Model file for the job. Use its own axes, mm. Face numbers are marked on the shaded views. A direction names the side the tool comes from. Round coordinates to 2 decimals unless told otherwise and drop trailing zeros. Loops run counter-clockwise (first coordinate to the right, second up) from the corner with the lowest first, then second, coordinate; pieces in that order, holes last. Notation, with made-up numbers: (66, -22) -> (118, -22) arc R22 cw to (118, 9) -> close; hole circle Ø5 at (20.5, 75.25). An arc over 180 degrees is marked (long way). Use a Markdown table: item, result.
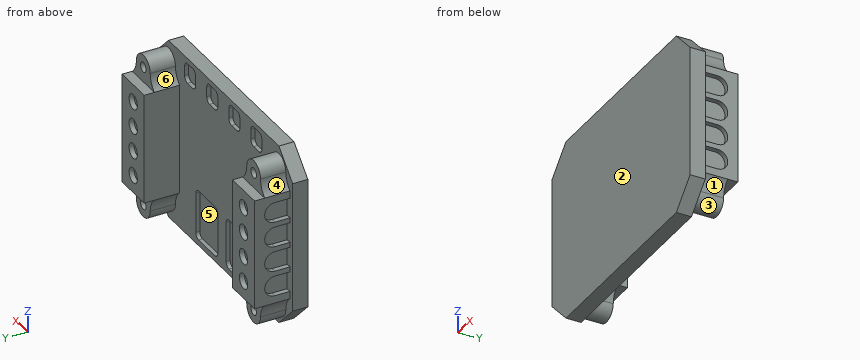
from build123d import *

# Parameters (mm, degrees)
SALIENTE_EXTRUIR1_DEPTH = 3
CROQUIS2_R              = 1
SALIENTE_EXTRUIR2_DEPTH = 7
CROQUIS3_W              = 8.584431172
CROQUIS3_H              = 6.245278734
CROQUIS3_W_2            = 9.103782271
CROQUIS3_H_2            = 6.523642819
CORTAR_EXTRUIR1_DEPTH   = 2
CROQUIS4_R              = 1.5
CORTAR_EXTRUIR2_DEPTH   = 1
CORTAR_EXTRUIR3_DEPTH   = 1
CORTAR_EXTRUIR4_DEPTH   = 0.8


with BuildPart() as part:
    # Croquis1 → Saliente-Extruir1 (new body)
    with BuildSketch(Plane(origin=(0, 0, 0), x_dir=(1, 0, 0), z_dir=(0, 1, 0))):
        Polygon((-25, -13), (-20, -18), (20, -18), (25, -13), (25, 13), (20, 18), (-20, 18), (-25, 13), align=None)
    extrude(amount=SALIENTE_EXTRUIR1_DEPTH)

    # Croquis2 → Saliente-Extruir2 (add)
    with BuildSketch(Plane(origin=(0, 3, 0), x_dir=(1, 0, 0), z_dir=(0, 1, 0))):
        with BuildLine():
            Line((-24, 11), (-24, -11))
            ThreePointArc((-24, -11), (-22.910217487, -12.356554061), (-22.499549169, -14.047475815))
            ThreePointArc((-22.499549169, -14.047475815), (-20, -16.5), (-17.500450831, -14.047475815))
            ThreePointArc((-17.500450831, -14.047475815), (-17.089782513, -12.356554061), (-16, -11))
            Line((-16, -11), (-16, 11))
            ThreePointArc((-16, 11), (-17.089782513, 12.356554061), (-17.500450831, 14.047475815))
            ThreePointArc((-17.500450831, 14.047475815), (-20, 16.5), (-22.499549169, 14.047475815))
            ThreePointArc((-22.499549169, 14.047475815), (-22.910217487, 12.356554061), (-24, 11))
        make_face()
        with Locations(Location((-20, -14, 0), (0, 0, 270))):
            Circle(CROQUIS2_R, mode=Mode.SUBTRACT)
        with Locations(Location((-20, 14, 0), (0, 0, 90))):
            Circle(CROQUIS2_R, mode=Mode.SUBTRACT)
    saliente_extruir2 = extrude(amount=SALIENTE_EXTRUIR2_DEPTH)

    # Croquis3 → Cortar-Extruir1 (cut)
    with BuildSketch(Plane(origin=(0, 10, 0), x_dir=(1, 0, 0), z_dir=(0, 1, 0))):
        with Locations((-19.707784414, -14.122639367)):
            Rectangle(CROQUIS3_W, CROQUIS3_H)
        with Locations((-20.551891136, 14.26182141)):
            Rectangle(CROQUIS3_W_2, CROQUIS3_H_2)
    cortar_extruir1 = extrude(amount=-CORTAR_EXTRUIR1_DEPTH, mode=Mode.SUBTRACT)

    # Croquis4 → Cortar-Extruir2 (cut)
    with BuildSketch(Plane(origin=(0, 10, 0), x_dir=(1, 0, 0), z_dir=(0, 1, 0))):
        with Locations(Location((-20, 7.5, 0), (0, 0, 270))):
            Circle(CROQUIS4_R)
        with Locations(Location((-20, 2.5, 0), (0, 0, 270))):
            Circle(CROQUIS4_R)
        with Locations(Location((-20, -2.5, 0), (0, 0, 270))):
            Circle(CROQUIS4_R)
        with Locations(Location((-20, -7.5, 0), (0, 0, 270))):
            Circle(CROQUIS4_R)
    cortar_extruir2 = extrude(amount=-CORTAR_EXTRUIR2_DEPTH, mode=Mode.SUBTRACT)

    # Croquis5 → Cortar-Extruir3 (cut)
    with BuildSketch(Plane.ZY.offset(24)):
        with BuildLine():
            Line((-9.5, 6), (-9.5, 3))
            Line((-9.5, 3), (-5.5, 3))
            Line((-5.5, 3), (-5.5, 6))
            ThreePointArc((-5.5, 6), (-7.5, 8), (-9.5, 6))
        make_face()
        with BuildLine():
            Line((-0.5, 3), (-0.5, 6))
            ThreePointArc((-0.5, 6), (-2.5, 8), (-4.5, 6))
            Line((-4.5, 6), (-4.5, 3))
            Line((-4.5, 3), (-0.5, 3))
        make_face()
        with BuildLine():
            Line((4.5, 3), (4.5, 6))
            ThreePointArc((4.5, 6), (2.5, 8), (0.5, 6))
            Line((0.5, 6), (0.5, 3))
            Line((0.5, 3), (4.5, 3))
        make_face()
        with BuildLine():
            Line((9.5, 3), (9.5, 6))
            ThreePointArc((9.5, 6), (7.5, 8), (5.5, 6))
            Line((5.5, 6), (5.5, 3))
            Line((5.5, 3), (9.5, 3))
        make_face()
    cortar_extruir3 = extrude(amount=-CORTAR_EXTRUIR3_DEPTH, mode=Mode.SUBTRACT)

    # Simetría1: Saliente-Extruir2, Cortar-Extruir1, Cortar-Extruir2, Cortar-Extruir3 across plane
    add(saliente_extruir2.mirror(Plane(origin=(0, 0, 0), x_dir=(0, 0, 1), z_dir=(1, 0, 0))))
    add(cortar_extruir1.mirror(Plane(origin=(0, 0, 0), x_dir=(0, 0, 1), z_dir=(1, 0, 0))), mode=Mode.SUBTRACT)
    add(cortar_extruir2.mirror(Plane(origin=(0, 0, 0), x_dir=(0, 0, 1), z_dir=(1, 0, 0))), mode=Mode.SUBTRACT)
    add(cortar_extruir3.mirror(Plane(origin=(0, 0, 0), x_dir=(0, 0, 1), z_dir=(1, 0, 0))), mode=Mode.SUBTRACT)

    # Croquis6 → Cortar-Extruir4 (cut)
    with BuildSketch(Plane(origin=(0, 3, 0), x_dir=(1, 0, 0), z_dir=(0, 1, 0))):
        with BuildLine():
            Line((-4.849514856, -12.944900329), (-2.849514856, -12.944900329))
            ThreePointArc((-2.849514856, -12.944900329), (-2.142408074, -13.237793547), (-1.849514856, -13.944900329))
            Line((-1.849514856, -13.944900329), (-1.849514856, -15.944900329))
            ThreePointArc((-1.849514856, -15.944900329), (-2.142408074, -16.65200711), (-2.849514856, -16.944900329))
            Line((-2.849514856, -16.944900329), (-4.849514856, -16.944900329))
            ThreePointArc((-4.849514856, -16.944900329), (-5.556621637, -16.65200711), (-5.849514856, -15.944900329))
            Line((-5.849514856, -15.944900329), (-5.849514856, -13.944900329))
            ThreePointArc((-5.849514856, -13.944900329), (-5.556621637, -13.237793547), (-4.849514856, -12.944900329))
        make_face()
        with BuildLine():
            Line((-7.889343155, 16.87305495), (-1.889343155, 16.87305495))
            ThreePointArc((-1.889343155, 16.87305495), (-1.182236374, 16.580161731), (-0.889343155, 15.87305495))
            Line((-0.889343155, 15.87305495), (-0.889343155, 7.87305495))
            ThreePointArc((-0.889343155, 7.87305495), (-1.182236374, 7.165948169), (-1.889343155, 6.87305495))
            Line((-1.889343155, 6.87305495), (-7.889343155, 6.87305495))
            ThreePointArc((-7.889343155, 6.87305495), (-8.596449936, 7.165948169), (-8.889343155, 7.87305495))
            Line((-8.889343155, 7.87305495), (-8.889343155, 15.87305495))
            ThreePointArc((-8.889343155, 15.87305495), (-8.596449936, 16.580161731), (-7.889343155, 16.87305495))
        make_face()
        with BuildLine():
            Line((3.130467216, 16.87305495), (9.130467216, 16.87305495))
            ThreePointArc((9.130467216, 16.87305495), (9.837573998, 16.580161731), (10.130467216, 15.87305495))
            Line((10.130467216, 15.87305495), (10.130467216, 7.87305495))
            ThreePointArc((10.130467216, 7.87305495), (9.837573998, 7.165948169), (9.130467216, 6.87305495))
            Line((9.130467216, 6.87305495), (3.130467216, 6.87305495))
            ThreePointArc((3.130467216, 6.87305495), (2.423360435, 7.165948169), (2.130467216, 7.87305495))
            Line((2.130467216, 7.87305495), (2.130467216, 15.87305495))
            ThreePointArc((2.130467216, 15.87305495), (2.423360435, 16.580161731), (3.130467216, 16.87305495))
        make_face()
        with BuildLine():
            Line((-12.849514856, -12.944900329), (-10.849514856, -12.944900329))
            ThreePointArc((-10.849514856, -12.944900329), (-10.142408074, -13.237793547), (-9.849514856, -13.944900329))
            Line((-9.849514856, -13.944900329), (-9.849514856, -15.944900329))
            ThreePointArc((-9.849514856, -15.944900329), (-10.142408074, -16.65200711), (-10.849514856, -16.944900329))
            Line((-10.849514856, -16.944900329), (-12.849514856, -16.944900329))
            ThreePointArc((-12.849514856, -16.944900329), (-13.556621637, -16.65200711), (-13.849514856, -15.944900329))
            Line((-13.849514856, -15.944900329), (-13.849514856, -13.944900329))
            ThreePointArc((-13.849514856, -13.944900329), (-13.556621637, -13.237793547), (-12.849514856, -12.944900329))
        make_face()
        with BuildLine():
            Line((3.150485144, -12.944900329), (5.150485144, -12.944900329))
            ThreePointArc((5.150485144, -12.944900329), (5.857591926, -13.237793547), (6.150485144, -13.944900329))
            Line((6.150485144, -13.944900329), (6.150485144, -15.944900329))
            ThreePointArc((6.150485144, -15.944900329), (5.857591926, -16.65200711), (5.150485144, -16.944900329))
            Line((5.150485144, -16.944900329), (3.150485144, -16.944900329))
            ThreePointArc((3.150485144, -16.944900329), (2.443378363, -16.65200711), (2.150485144, -15.944900329))
            Line((2.150485144, -15.944900329), (2.150485144, -13.944900329))
            ThreePointArc((2.150485144, -13.944900329), (2.443378363, -13.237793547), (3.150485144, -12.944900329))
        make_face()
        with BuildLine():
            Line((11.150485144, -12.944900329), (13.150485144, -12.944900329))
            ThreePointArc((13.150485144, -12.944900329), (13.857591926, -13.237793547), (14.150485144, -13.944900329))
            Line((14.150485144, -13.944900329), (14.150485144, -15.944900329))
            ThreePointArc((14.150485144, -15.944900329), (13.857591926, -16.65200711), (13.150485144, -16.944900329))
            Line((13.150485144, -16.944900329), (11.150485144, -16.944900329))
            ThreePointArc((11.150485144, -16.944900329), (10.443378363, -16.65200711), (10.150485144, -15.944900329))
            Line((10.150485144, -15.944900329), (10.150485144, -13.944900329))
            ThreePointArc((10.150485144, -13.944900329), (10.443378363, -13.237793547), (11.150485144, -12.944900329))
        make_face()
    extrude(amount=-CORTAR_EXTRUIR4_DEPTH, mode=Mode.SUBTRACT)


solid = part.part
Q1. Flat gauge pins, fed straight in: pin 1 (1.1 mm diameter, centred on x = 23.5, y = 5, fed in from +Z); pin 2 (1.6 mm diameter, centred on x = 20, z = -13.5, fed in from +Y); pin 3 (6 mm diameter, centred on x = 3, z = 5, fed in from +Y). Where does each tip first touch, or does it go through?
Results list:
| item | result |
|---|---|
| pin 1 | stops at z = 12.28 |
| pin 2 | stops at y = 8 |
| pin 3 | stops at y = 3 |
Q2. Tool access for the marked faces 4, 5 and 6: list every direction of +Z, -Z, +X, -X, +Y, -Y with a clear straight run to the whole face (end or side of a thin tool).
Results list:
| item | result |
|---|---|
| face 4 | +Z, -X, +Y |
| face 5 | +Y |
| face 6 | +Z, +Y |
Q3. Pull direction X, two halves, no side cores. Call the marked faces 1, 2 and 3: released by +X, released by -X, zero draft, split by the parting line, or undercut.
Results list:
| item | result |
|---|---|
| face 1 | released by +X |
| face 2 | zero draft |
| face 3 | undercut |
Q4. Band-saw the part on C-C, the plane y = 7. Give the number of separate pieces and of enclosed holes in the cut face, plus the area to 3 significant figures.
Results list:
| item | result |
|---|---|
| separate pieces | 2 |
| enclosed holes | 4 |
| area | 422 mm² |
Q5. Drill centre lines: L1, parallel to Z at x = -20, y = 6.05; L2, parallel to X at y = 4.1, z = 14; L3, parallel to X at y = 9.45, z = 7.5. Where is each one in solid material? Low to high. Write a range as from..to.
Results list:
| item | result |
|---|---|
| L1 | z = -16.5..-15, -13..13, 15..16.5 |
| L2 | x = -22.5..-21, -19..-17.5, 17.5..19, 21..22.5 |
| L3 | x = -24..-21.5, -18.5..-16, 16..18.5, 21.5..24 |
Q6. Band-saw the part on B-B, the plane z = 7.5. Give the cut face in (x, y).
Results list:
| item | result |
|---|---|
| outline | (-25, 0) -> (25, 0) -> (25, 3) -> (23, 3) -> (23, 8) -> (24, 8) -> (24, 10) -> (21.5, 10) -> (21.5, 9) -> (18.5, 9) -> (18.5, 10) -> (16, 10) -> (16, 3) -> (-16, 3) -> (-16, 10) -> (-18.5, 10) -> (-18.5, 9) -> (-21.5, 9) -> (-21.5, 10) -> (-24, 10) -> (-24, 8) -> (-23, 8) -> (-23, 3) -> (-25, 3) -> close |
Q7. Band-saw the part on A-A, the plane x = 7. Give the cut face in (y, z), plus the area to 3 significant figures.
Results list:
| item | result |
|---|---|
| outline | (0, -18) -> (3, -18) -> (3, -16.87) -> (2.2, -16.87) -> (2.2, -6.87) -> (3, -6.87) -> (3, 18) -> (0, 18) -> close |
| area | 100 mm² |
Q8. Band-saw the part on D-D, the plane x = -15. Give the cut face in (y, z), plus the area to 3 significant figures.
Results list:
| item | result |
|---|---|
| outline | (0, -18) -> (3, -18) -> (3, 18) -> (0, 18) -> close |
| area | 108 mm² |
